from build123d import *

# Parameters (mm, degrees)
SKETCH1_W           = 2
SKETCH1_H           = 5
SKETCH1_W_2         = 5
SKETCH1_H_2         = 2
BOSS_EXTRUDE1_DEPTH = 2


with BuildPart() as part:
    # Sketch1 → Boss-Extrude1 (new body)
    with BuildSketch(Plane(origin=(0, 0, 0), x_dir=(1, 0, 0), z_dir=(0, 1, 0))):
        Polygon((10, 0), (0, 10), (0, 0), align=None)
        with Locations((-1, 7.5)):
            Rectangle(SKETCH1_W, SKETCH1_H)
        with Locations((7.5, -1)):
            Rectangle(SKETCH1_W_2, SKETCH1_H_2)
    extrude(amount=BOSS_EXTRUDE1_DEPTH)


solid = part.part
Input: part model. Units: mm. Frame: model coordinates. A direction names the side the tool comes from. Coordinates: 2 decimals unless noted, no trailing zeros. Order: outer loops, then holes, each group sorted by start corner. A loop starts at its lowest first (then second) coordinate and runs counter-clockwise, first axis right, second up. Notation, with made-up numbers: M 69.5,-6 L 97.5,-6 A13 cw 97.5,15 Z; hole C 70.25,80 d7. An arc over 180 degrees is marked long. Write item = value, one per line. Start each with the question number.
(1) First-contact query: P1, Ø1, axis at y = 0.5, z = -1.5, coming from the -X side; P2, Ø1, axis at x = 3, y = 1, coming from the +Z side; P3, Ø0.6, axis at y = 1, z = 0.5, coming from the -X side. Flat tips, straight axial feed; report the tip coordinate or a pass-through.
(2) Section C-C on z = -7. Output: boundary loops of the cut face in (x, y).
(3) Reachability of faces 1 (the flat face through (-1, 1, -5)), 2 (the flat face through (4, 2, -3)) from +Z, -Z, +X, -X, +Y, -Y: full face, straight path, thin tool, end or side. Return the list, or none.
(4) Section B-B on x = 0.25. Output: boundary loops of the cut face in (y, z), and give its area (3 significant figures).
(5) Line query: line 1 along X through (y, z) = (1.75, 0.25); line 2 along Z through (x, y) = (6, 1.05); line 3 along X through (y, z) = (0.9, -9). Output: solid intervals per line, ascending. Write a range as [from, to].
(6) Section A-A on y = 0.5. Output: boundary loops of the cut face in (x, z), and give its area (3 significant figures).
Result set:
q1.P1 = 0
q1.P2 = 0
q1.P3 = 5
q2.outline = M -2,0 L 3,0 L 3,2 L -2,2 Z
q3.face_1 = +Z, -X, +Y, -Y
q3.face_2 = +Z, -Z, +X, -X, +Y
q4.outline = M 0,-9.75 L 2,-9.75 L 2,0 L 0,0 Z
q4.area = 19.5 mm²
q5.line_1 = [5, 10]
q5.line_2 = [-4, 2]
q5.line_3 = [-2, 1]
q6.outline = M -2,-10 L 0,-10 L 10,0 L 10,2 L 5,2 L 5,0 L 0,0 L 0,-5 L -2,-5 Z
q6.area = 70.0 mm²
